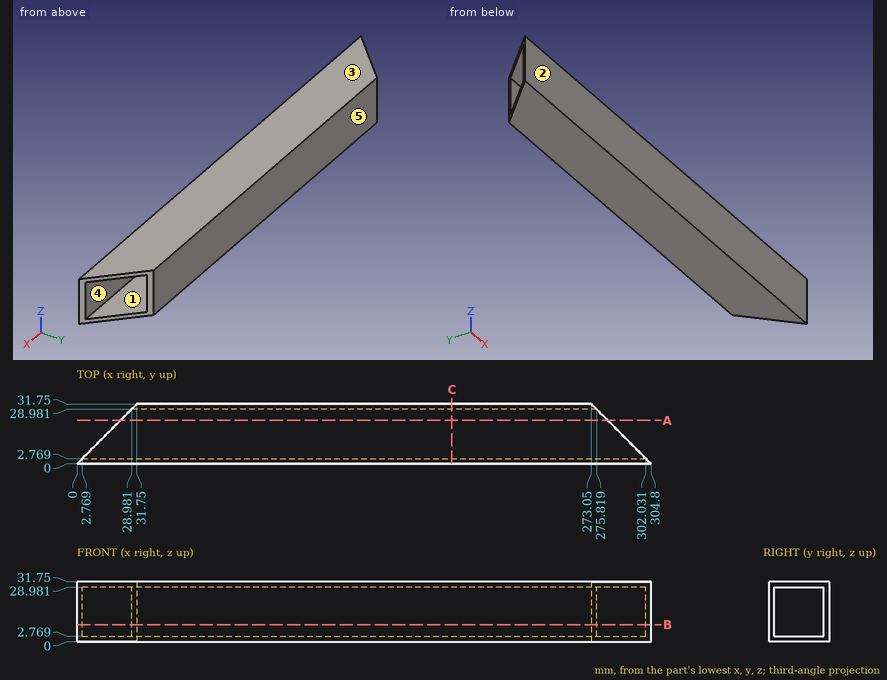
Print and shaded views of the part. All mm, measured from the part's lowest x, y and z. A direction names the side the tool comes from. Give positions to 0.01 mm unless a question says otherwise; leave off trailing zeros. Loops run counter-clockwise (first coordinate to the right, second up) from the corner with the lowest first, then second, coordinate; pieces in that order, holes last. Notation, with made-up numbers: (73.25, -6) - (109.25, -6) arc R13 ccw to (109.25, -1) - close; hole circle Ø6 at (11.25, 41). An arc over 180 degrees is marked (long way). One line per item, written item: value. Start each with the question number.
1. Pull direction Z, two halves, no side cores. Call the marked faces 1, 2 and 3: pulls with the +Z half, pulls with the -Z half, needs draft (parallel to the pull), parting line crosses it, or undercut.
2. Slice it at C-C (x = 199). List the corners of the cut face in (y, z).
3. Slice it at A-A (y = 23). List the corners of the cut face in (x, z).
4. Slice it at B-B (z = 9). List the corners of the cut face in (x, y).
5. Probe L1, parallel to Z at x = 223, y = 26; L2, parallel to X at y = 1, z = 9. List the from-to ranges inside material, lowest first. Write a range as from..to.
6. Which spindle directions (+Z, -Z, +X, -X, +Y, -Y) get a long thin tool onto all of the face, cutting with end or side? Do the marked faces 4 and 5. Say none if no direction does.
Solution:
1. face 1: undercut
1. face 2: needs draft
1. face 3: pulls with the +Z half
2. outline: (0, 0) - (31.75, 0) - (31.75, 31.75) - (0, 31.75) - close; hole (2.77, 2.77) - (28.98, 2.77) - (28.98, 28.98) - (2.77, 28.98) - close
3. outline: (23, 0) - (281.8, 0) - (281.8, 2.77) - (23, 2.77) - close; (23, 28.98) - (281.8, 28.98) - (281.8, 31.75) - (23, 31.75) - close
4. outline: (0, 0) - (304.8, 0) - (302.03, 2.77) - (2.77, 2.77) - close; (28.98, 28.98) - (275.82, 28.98) - (273.05, 31.75) - (31.75, 31.75) - close
5. L1: z = 0..2.77, 28.98..31.75
5. L2: x = 1..303.8
6. face 4: +X, -X
6. face 5: +Z, -Z, +X, -X, +Y
